from build123d import *

# Parameters (mm, degrees)
F0_R          = 10
F1_DEPTH      = 1
F3_W          = 26
F3_H          = 5
F4_DEPTH      = 1
F5_R          = 3.85
F5_R_2        = 2.85
F7_DEPTH      = 6
F6_R          = 2.85
F8_DEPTH      = 6.001
F8_DEPTH_BACK = 1.001


with BuildPart() as f1:
    # F0 (on Front) → F1 (new body)
    with BuildSketch(Plane.XZ):
        Circle(F0_R)
    extrude(amount=F1_DEPTH)

    # F3 (on face) → F4 (join)
    with BuildSketch(Plane(origin=(0, 0, 0), x_dir=(-1, 0, 0), z_dir=(0, 1, 0))):
        Rectangle(F3_W, F3_H)
    extrude(amount=-F4_DEPTH)

    # F5 (on face) → F7 (join)
    with BuildSketch(Plane.XZ.offset(1)):
        Circle(F5_R)
        Circle(F5_R_2, mode=Mode.SUBTRACT)
    extrude(amount=F7_DEPTH)

    # F6 (on face) → F8 (cut, two sides)
    with BuildSketch(Plane.XZ.offset(1)) as f8_sk:
        Circle(F6_R)
    extrude(amount=F8_DEPTH, mode=Mode.SUBTRACT)
    extrude(f8_sk.sketch, amount=-F8_DEPTH_BACK, mode=Mode.SUBTRACT)


solid = f1.part
The listing builds one solid part. Answer for the finished solid, in the listing's coordinates (mm). A direction names the side the tool comes from. Give positions to 0.01 mm unless a question says otherwise; leave off trailing zeros. Loops run counter-clockwise (first coordinate to the right, second up) from the corner with the lowest first, then second, coordinate; pieces in that order, holes last. Notation, with made-up numbers: (16, -21.75) - (36, -21.75) arc R22 cw to (36, 15.25) - close; hole circle Ø9 at (-11, 38). An arc over 180 degrees is marked (long way). Write each question's results on one line, items separated by ' | '.
1. Find section D-D, the plane x = -3.5. Write down the section's boundary in (y, z), then the cut area to 3 significant figures.
Resolved:
outline: (-7, -1.6) - (-1, -1.6) - (-1, -9.37) - (0, -9.37) - (0, 9.37) - (-1, 9.37) - (-1, 1.6) - (-7, 1.6) - close | area: 38.0 mm^2
2. Which of the six approach directions +Z, -Z, +X, -X, +Y, -Y give full straight-line access (tool end or side, diameter ignored) to faces 1 (the face through (11.4, -0.5, -2.5)), 2 (the face through (-11.3, -0.5, 2.5)), 3 (the face through (11.4, -0.5, 2.5)), 4 (the face through (0, -1, 5))?
Resolved:
face 1: -Z, +X, +Y, -Y | face 2: +Z, -X, +Y, -Y | face 3: +Z, +X, +Y, -Y | face 4: -Y
3. Find section A-A, the plane z = 0. Write down the section's boundary in (x, y), then the cut area to 3 significant figures.
Resolved:
outline: (-13, -1) - (-3.85, -1) - (-3.85, -7) - (-2.85, -7) - (-2.85, 0) - (-13, 0) - close; (2.85, -7) - (3.85, -7) - (3.85, -1) - (13, -1) - (13, 0) - (2.85, 0) - close | area: 32.3 mm^2
4. Find section C-C, the plane y = -1.75. Write down the section's boundary in (x, z), then the cut area to 3 significant figures.
Resolved:
outline: circle Ø7.7 at (0, 0); hole circle Ø5.7 at (0, 0) | area: 21.0 mm^2
5. Flat-ended cylindrical pins translate along their axes: P1, Ø3.5, axis at x = 0, z = 0, coming from the +Y side; P2, Ø4, axis at y = -5, z = -4.5, coming from the -X side; P3, Ø0.8, axis at x = 11, y = -0.5, coming from the +Z side; P4, Ø1.1, axis at x = 10.5, y = -0.5, coming from the -Z side. Find the tip coordinate at first contact, or state that the pin passes through.
Resolved:
P1: passes through | P2: stops at x = -2.93 | P3: stops at z = 2.5 | P4: stops at z = -2.5
6. Find section B-B, the plane x = 0. Write down the section's boundary in (y, z).
Resolved:
outline: (-7, -3.85) - (-1, -3.85) - (-1, -10) - (0, -10) - (0, -2.85) - (-7, -2.85) - close; (-7, 2.85) - (0, 2.85) - (0, 10) - (-1, 10) - (-1, 3.85) - (-7, 3.85) - close
7. Consider probe 1 along Z at (x, y) = (0, -4.3); probe 2 along Z at (x, y) = (0, -0.3); probe 3 along Y at (x, z) = (-9.5, 0.5). Determine where each line is inside the solid, lowest interval first. Write a range as from..to.
Resolved:
probe 1: z = -3.85..-2.85, 2.85..3.85 | probe 2: z = -10..-2.85, 2.85..10 | probe 3: y = -1..0
